Build history of the part. All positions in model axes, mm. Face numbers are marked on the shaded views. A direction names the side the tool comes from. Round coordinates to 2 decimals unless told otherwise and drop trailing zeros. Loops run counter-clockwise (first coordinate to the right, second up) from the corner with the lowest first, then second, coordinate; pieces in that order, holes last. Notation, with made-up numbers: (64, 25) - (84, 25) arc R29 cw to (84, 50) - close; hole circle Ø10 at (63, 72.5). An arc over 180 degrees is marked (long way). Use a Markdown table: item, result.
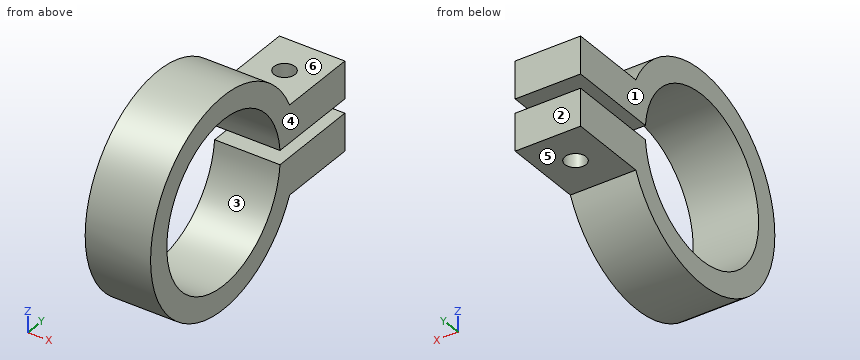
from build123d import *

# Parameters (mm, degrees)
F1_DEPTH = 14
F3_D     = 4.5


with BuildPart() as f1:
    # F0 (on Right) → F1 (new body)
    with BuildSketch(Plane.YZ):
        with BuildLine():
            ThreePointArc((17.4355957742, -1.5), (-17.5, 0), (17.4355957742, 1.5))
            Line((17.4355957742, 1.5), (37.4355957742, 1.5))
            Line((37.4355957742, 1.5), (37.4355957742, 9.5))
            Line((37.4355957742, 9.5), (20.3960780544, 9.5))
            ThreePointArc((20.3960780544, 9.5), (-14.6168366424, 17.1054987232), (-12.5644042258, -18.6650943327))
            ThreePointArc((-12.5644042258, -18.6650943327), (6.027729031, -21.6775571209), (20.3960780544, -9.5))
            Line((20.3960780544, -9.5), (37.4355957742, -9.5))
            Line((37.4355957742, -9.5), (37.4355957742, -1.5))
            Line((37.4355957742, -1.5), (17.4355957742, -1.5))
        make_face()
    extrude(amount=F1_DEPTH)

    # F3 (through all)
    with Locations(Plane.XY.offset(9.5)):
        with Locations((7, 28.9158369143)):
            Hole(F3_D / 2)


solid = f1.part
Q1. Cut at A-A, the plane y = 0. List the corners of the cut face in (x, z), plus the area to 3 significant figures.
Results found:
| item | result |
|---|---|
| outline | (0, -22.5) - (14, -22.5) - (14, -17.5) - (0, -17.5) - close; (0, 17.5) - (14, 17.5) - (14, 22.5) - (0, 22.5) - close |
| area | 140 mm2 |
Q2. Probe line 1 (Z direction, x = 11.25, y = 34); line 2 (Z direction, x = 8.75, y = 0); line 3 (Y direction, x = 7, z = 3.25). List the from-to ranges inside material, lowest first.
Results found:
| item | result |
|---|---|
| line 1 | z = -9.5 to -1.5, 1.5 to 9.5 |
| line 2 | z = -22.5 to -17.5, 17.5 to 22.5 |
| line 3 | y = -22.26 to -17.2, 17.2 to 26.67, 31.17 to 37.44 |
Q3. Drop flat-ended pins along their axis: pin 1 (5 mm diameter, centred on x = 7, y = 28.92, fed in from -Z); pin 2 (21 mm diameter, centred on y = 0, z = 0, fed in from +X); pin 3 (6 mm diameter, centred on x = 8, y = 14.5, fed in from -Z); pin 4 (3 mm diameter, centred on x = 8, z = -7.5, fed in from -Y). Give the stop position or say it passes through.
Results found:
| item | result |
|---|---|
| pin 1 | stops at z = -9.5 |
| pin 2 | passes through |
| pin 3 | stops at z = -19.34 |
| pin 4 | stops at y = -21.69 |
Q4. Which spindle directions (+Z, -Z, +X, -X, +Y, -Y) get a long thin tool onto all of the face, cutting with end or side? Do the marked faces 4, 5 and 6. Say none if no direction does.
Results found:
| item | result |
|---|---|
| face 4 | +Z, -Z, +X, +Y, -Y |
| face 5 | -Z, +X, -X, +Y |
| face 6 | +Z, +X, -X, +Y |
Q5. Cut at D-D, the plane x = 12.5. List the corners of the cut face in (y, z).
Results found:
| item | result |
|---|---|
| outline | (17.44, -1.5) arc R17.5 cw (long way) to (17.44, 1.5) - (37.44, 1.5) - (37.44, 9.5) - (20.4, 9.5) arc R22.5 ccw (long way) to (20.4, -9.5) - (37.44, -9.5) - (37.44, -1.5) - close |
Q6. Cut at B-B, the plane x = 7. List the corners of the cut face in (y, z), plus the area to 3 significant figures.
Results found:
| item | result |
|---|---|
| outline | (17.44, -1.5) arc R17.5 cw (long way) to (17.44, 1.5) - (26.67, 1.5) - (26.67, 9.5) - (20.4, 9.5) arc R22.5 ccw (long way) to (20.4, -9.5) - (26.67, -9.5) - (26.67, -1.5) - close; (31.17, -9.5) - (37.44, -9.5) - (37.44, -1.5) - (31.17, -1.5) - close; (31.17, 1.5) - (37.44, 1.5) - (37.44, 9.5) - (31.17, 9.5) - close |
| area | 793 mm2 |
Q7. Cut at C-C, the plane z = -5. List the corners of the cut face in (x, y).
Results found:
| item | result |
|---|---|
| outline | (0, -21.94) - (14, -21.94) - (14, -16.77) - (0, -16.77) - close; (0, 16.77) - (14, 16.77) - (14, 37.44) - (0, 37.44) - close; hole circle Ø4.5 at (7, 28.92) |
Q8. Pull direction Y, two halves, no side cores. Call the marked faces 1, 2 and 3: pulls with the +Y half, pulls with the -Y half, needs draft (parallel to the pull), parting line crosses it, or undercut.
Results found:
| item | result |
|---|---|
| face 1 | needs draft |
| face 2 | pulls with the +Y half |
| face 3 | undercut |
